```python
from build123d import *

# Parameters (mm, degrees)
F1_DEPTH = 25.4
F3_DEPTH = 25.4
F5_DEPTH = 25.4
F7_DEPTH = 25.4
F8_R     = 5.84435
F8_R_2   = 5.993936
F9_DEPTH = 25.4


with BuildPart() as f1:
    # F0 (on Front) → F1 (new body)
    with BuildSketch(Plane.XZ):
        Polygon((-70.167482, 32.861239), (-70.167482, 0), (-19.367482, 0), (-19.367482, 12.7), (-57.467482, 12.7), (-57.467482, 32.861239), align=None)
    extrude(amount=F1_DEPTH)

    # F2 (on face) → F3 (cut)
    with BuildSketch(Plane.YZ.offset(-57.467482)):
        with BuildLine():
            ThreePointArc((-25.4, 22.78062), (-12.7, 31.897256), (0, 22.78062))
            Line((0, 22.78062), (0, 32.861239))
            Line((0, 32.861239), (-25.4, 32.861239))
            Line((-25.4, 32.861239), (-25.4, 22.78062))
        make_face()
    extrude(amount=-F3_DEPTH, mode=Mode.SUBTRACT)

    # F4 (on face) → F5 (cut)
    with BuildSketch(Plane.YZ.offset(-57.467482)):
        with BuildLine():
            ThreePointArc((-20.083626, 22.106148), (-13.406311, 28.783463), (-6.728996, 22.106148))
            Line((-6.728996, 22.106148), (-6.728996, 30.493881))
            ThreePointArc((-6.728996, 30.493881), (-13.515075, 31.872452), (-20.083626, 29.680317))
            Line((-20.083626, 29.680317), (-20.083626, 22.106148))
        make_face()
        with BuildLine():
            ThreePointArc((-20.083626, 22.106148), (-13.406311, 15.428833), (-6.728996, 22.106148))
            ThreePointArc((-6.728996, 22.106148), (-13.406311, 28.783463), (-20.083626, 22.106148))
        make_face()
    extrude(amount=-F5_DEPTH, mode=Mode.SUBTRACT)

    # F6 (on face) → F7 (cut)
    with BuildSketch(Plane.XY.offset(12.7)):
        with BuildLine():
            ThreePointArc((-28.238824, 0), (-19.601071, -13.225048), (-29.665027, -25.4))
            Line((-29.665027, -25.4), (-19.367482, -25.4))
            Line((-19.367482, -25.4), (-19.367482, 0))
            Line((-19.367482, 0), (-28.238824, 0))
        make_face()
    extrude(amount=-F7_DEPTH, mode=Mode.SUBTRACT)

    # F8 (on face) → F9 (cut)
    with BuildSketch(Plane.XY.offset(12.7)):
        with Locations((-32.900844, -12.478269)):
            Circle(F8_R)
        with Locations((-49.631871, -12.7)):
            Circle(F8_R_2)
    extrude(amount=-F9_DEPTH, mode=Mode.SUBTRACT)


solid = f1.part
```
Model file for the job. Use its own axes, mm. A direction names the side the tool comes from. Coordinates: 2 decimals unless noted, no trailing zeros. Order: outer loops, then holes, each group sorted by start corner. A loop starts at its lowest first (then second) coordinate and runs counter-clockwise, first axis right, second up. Notation, with made-up numbers: (-37.75, 35) -> (18.25, 35) arc R16 cw to (18.25, 42) -> close; hole circle Ø3 at (61, 40.25). An arc over 180 degrees is marked (long way). Return JSON: item names as keys, results as strings.
Item 1: 3-axis set-ups, long thin cutter, end or side, ignore diameter. For faces 5 (the face through (-44.095, -14.996, 6.439)), 6 (the face through (-64, -20.084, 26)), 7 (the face through (-38.3, -15.3, 12.7)): which of +Z, -Z, +X, -X, +Y, -Y reach the whole face in a straight line?
Model answer:
{"face 5": "+Z, -Z", "face 6": "+Z, +X, -X", "face 7": "+Z, +X, +Y, -Y"}
Item 2: Wall check: line 1 along X through (y, z) = (-15.25, 12); line 2 along Z through (x, y) = (-45, -2); line 3 along X through (y, z) = (-6.5, 17). Give the ranges that are in metal, low to high. Write a range as from..to.
Model answer:
{"line 1": "x = -70.17..-55.06, -44.21..-38.05, -27.76..-19.87", "line 2": "z = 0..12.7", "line 3": "x = -70.17..-57.47"}
Item 3: Slice it at B-B (z = 26.5). Write the cut outline in (x, y), then the cut area to 3 significant figures.
Model answer:
{"outline": "(-70.17, -23.45) -> (-57.47, -23.45) -> (-57.47, -20.08) -> (-70.17, -20.08) -> close; (-70.17, -6.73) -> (-57.47, -6.73) -> (-57.47, -1.95) -> (-70.17, -1.95) -> close", "area": "103 mm²"}
Item 4: Mould opens along Y. For faces 1 (the face through (-63.729, -23.356, 26.625)), 2 (the face through (-70.167, -13, 12)), 3 (the face through (-54, 0, 9)), 4 (the face through (-64, -6.729, 26)) say: pulls with the +Y half, pulls with the -Y half, needs draft (parallel to the pull), parting line crosses it, or undercut.
Model answer:
{"face 1": "pulls with the -Y half", "face 2": "needs draft", "face 3": "pulls with the +Y half", "face 4": "undercut"}
Item 5: Slice it at D-D (y = -5.25). Write the cut outline in (x, z).
Model answer:
{"outline": "(-70.17, 0) -> (-21.71, 0) -> (-21.71, 12.7) -> (-57.47, 12.7) -> (-57.47, 29.64) -> (-70.17, 29.64) -> close"}
Item 6: Slice it at C-C (x = -51.5). Write the cut outline in (y, z).
Model answer:
{"outline": "(-25.4, 0) -> (-18.4, 0) -> (-18.4, 12.7) -> (-25.4, 12.7) -> close; (-7, 0) -> (0, 0) -> (0, 12.7) -> (-7, 12.7) -> close"}
Item 7: Pin check, flat tips, straight feed: P1, Ø10, axis at x = -47.5, y = -6.5, coming from the -Z side; P2, Ø12, axis at y = -5.5, z = 26, coming from the +X side; P3, Ø5, axis at x = -27, y = -13, coming from the +Z side. Stop position of each tip, or through.
Model answer:
{"P1": "stops at z = 0", "P2": "stops at x = -57.47", "P3": "stops at z = 12.7"}
